Autodesk Inventor part; units mm, degrees
ref_plane "YZ Plane" through (0, 0, 0) normal (1, 0, 0) x (0, 1, 0)
ref_plane "XZ Plane" through (0, 0, 0) normal (0, 1, 0) x (-1, 0, 0)
ref_plane "XY Plane" through (0, 0, 0) normal (0, 0, 1) x (1, 0, 0)
sketch "Sketch1" plane through (0, 0, 0) normal (0, 0, 1) x (1, 0, 0)
  line L0 (12.5, -19) -> (-12.5, -19)
  line L1 (-12.5, -19) -> (-12.5, 19)
  line L2 (-12.5, 19) -> (12.5, 19)
  line L3 (12.5, 19) -> (12.5, -19)
  line L4 (12.5, -19) -> (-12.5, 19) construction
  line L5 (-12.5, -19) -> (12.5, 19) construction
  circle A0 centre (0, 12.5) radius 2.1
  circle A1 centre (0, -12.5) radius 2.1
  point P0 (0, 0)
  dimension "d0" = 25
  dimension "d1" = 38
  dimension "d2" = 4.2
  dimension "d3" = 4.2
  dimension "d4" = 12.5
  dimension "d5" = 12.5
extrude "Extrusion1" add sketch "Sketch1" along normal blind 40
sketch "Sketch2" plane through (-12.5, 19, 0) normal (0, 1, 0) x (1, 0, 0)
  line L0 (0, 0) -> (0, -40)
  line L1 (0, -40) -> (-6.5, -40)
  line L2 (-6.5, -40) -> (0, 0)
  line L3 (0, -40) -> (25, -40)
  line L4 (0, 0) -> (0, -40)
  line L5 (25, -40) -> (31.5, -40)
  line L6 (25, 0) -> (25, -40)
  line L7 (31.5, -40) -> (25, 0)
  line L8 (25, 0) -> (25, -40)
  point P0 (12.5, 0)
  dimension "d8" = 6.5
  dimension "d9" = 6.5
extrude "Extrusion2" add sketch "Sketch2" against normal up to surface (38 mm away)
sketch "Sketch3" plane through (0, 0, 40) normal (0, 0, 1) x (1, 0, 0)
  line L0 (-5.4088, 0) -> (7.7062, 0)
  line L1 (0, 5.8117) -> (0, -6.6687)
  point P0 (0, 0)
  point P1 (-16, 16)
  point P2 (16, 16)
  point P3 (-16, -16)
  point P4 (16, -16)
  dimension "d12" = 16
  dimension "d13" = 16
  dimension "d16" = 32
  dimension "d19" = 32
hole "Hole1" at (-16, 16, 40) at (16, 16, 40) at (-16, -16, 40) at (16, -16, 40) direction (0, 0, -1) diameter 2.5 end through all
hole "Hole2" at (0, -12.5, 40) direction (0, 0, -1) diameter 8 depth 36 tip angle 118
hole "Hole3" at (0, 12.5, 40) direction (0, 0, -1) diameter 8 depth 36 tip angle 118
properties part number "RDtoRC2-height40mm"
Design review of the part built by this model. Coordinates are the model's own, in mm. A direction names the side the tool comes from. Round coordinates to 2 decimals unless told otherwise and drop trailing zeros. Write each loop counter-clockwise with the first axis right and the second up, starting at its lowest first coordinate (ties: lowest second). Pieces come first, ordered by that corner, then holes. Notation, with made-up numbers: (36, -25.75) - (90, -25.75) arc R12 ccw to (90, -19.75) - close; hole circle Ø7 at (-2, 8.5). An arc over 180 degrees is marked (long way). Use a Markdown table: item, result. Add a question column.
1. We need section C-C (x = 16). State the section outline as (y, z) points.
2. Clearance check with flat-ended pins moving along their axes: pin 1 (6.5 mm diameter, centred on x = 0, y = -12.5, fed in from +Z); pin 2 (5 mm diameter, centred on x = 10, y = -11.5, fed in from -Z); pin 3 (1.5 mm diameter, centred on x = 16, y = 16, fed in from -Z); pin 4 (1.5 mm diameter, centred on y = -13, z = 5.5, fed in from +X). State where each tip first meets the part, or that it passes through.
3. Wall thickness on probe 1 along Y at (x, z) = (0, 24); probe 2 along Y at (x, z) = (0, 0.8); probe 3 along X at (y, z) = (-16, 28.25): over which ranges is each line inside the solid? List them lowest first.
4. We need section B-B (z = 31). State the section outline as (x, y) points, then the cut area to 3 significant figures.
5. We need section A-A (y = -12.5). State the section outline as (x, z) points, then the cut area to 3 significant figures.
6. For faces 1 (the face through (-0.273, 10.418, 1.409)), 2 (the face through (2.4, -9.3, 21.7)), list the 3-axis set-ups (+Z, -Z, +X, -X, +Y, -Y) from which the entire face can be reached by the end or side of a thin tool; tool diameter is ignored.
7. We need section D-D (z = 14.5). State the section outline as (x, y) points.
8. Mouldability with a two-part tool opening along Y and no side actions: class faces 3 (the face through (0, 19, 20)), 4 (the face through (-14.78, 16.27, 29.64)), 5 (the face through (0, -19, 20)) as +Y half, -Y half, draft (parallel to the pull), parting line (faces both ways), or undercut.
Output:
| question | item | result |
|---|---|---|
| 1 | outline | (-19, 21.54) - (-17.25, 21.54) - (-17.25, 40) - (-19, 40) - close; (-14.75, 21.54) - (14.75, 21.54) - (14.75, 40) - (-14.75, 40) - close; (17.25, 21.54) - (19, 21.54) - (19, 40) - (17.25, 40) - close |
| 2 | pin 1 | stops at z = 3.55 |
| 2 | pin 2 | stops at z = 0 |
| 2 | pin 3 | passes through |
| 2 | pin 4 | stops at x = 13.52 |
| 3 | probe 1 | y = -19 to -16.5, -8.5 to 8.5, 16.5 to 19 |
| 3 | probe 2 | y = -19 to -14.6, -10.4 to 10.4, 14.6 to 19 |
| 3 | probe 3 | x = -14.75 to -1.94, 1.94 to 14.75 |
| 4 | outline | (-17.54, -19) - (17.54, -19) - (17.54, 19) - (-17.54, 19) - close; hole circle Ø2.5 at (-16, -16); hole circle Ø2.5 at (-16, 16); hole circle Ø8 at (0, -12.5); hole circle Ø8 at (0, 12.5); hole circle Ø2.5 at (16, -16); hole circle Ø2.5 at (16, 16) |
| 4 | area | 1,210 mm2 |
| 5 | outline | (-19, 40) - (-12.5, 0) - (-2.1, 0) - (-2.1, 2.86) - (-4, 4) - (-4, 40) - close; (2.1, 0) - (12.5, 0) - (19, 40) - (4, 40) - (4, 4) - (2.1, 2.86) - close |
| 5 | area | 953 mm2 |
| 6 | face 1 | +Z, -Z |
| 6 | face 2 | +Z |
| 7 | outline | (-14.86, -19) - (14.86, -19) - (14.86, -16.5) arc R1.25 cw to (14.86, -15.5) - (14.86, 15.5) arc R1.25 cw to (14.86, 16.5) - (14.86, 19) - (-14.86, 19) - (-14.86, 16.5) arc R1.25 cw to (-14.86, 15.5) - (-14.86, -15.5) arc R1.25 cw to (-14.86, -16.5) - close; hole circle Ø8 at (0, -12.5); hole circle Ø8 at (0, 12.5) |
| 8 | face 3 | +Y half |
| 8 | face 4 | undercut |
| 8 | face 5 | -Y half |
